Work out the finished part from the listing and answer in its coordinate system (mm). A direction names the side the tool comes from. Coordinates: 2 decimals unless noted, no trailing zeros. Loops run counter-clockwise (first coordinate to the right, second up) from the corner with the lowest first, then second, coordinate; pieces in that order, holes last. Notation, with made-up numbers: (-17, 37.5) -> (38, 37.5) arc R24 ccw to (38, 60.5) -> close; hole circle Ø11 at (23.25, -28.5). An arc over 180 degrees is marked (long way). Use a Markdown table: item, result.
Autodesk Inventor part; units mm, degrees
ref_plane "YZ Plane" through (0, 0, 0) normal (1, 0, 0) x (0, 1, 0)
ref_plane "XZ Plane" through (0, 0, 0) normal (0, 1, 0) x (-1, 0, 0)
ref_plane "XY Plane" through (0, 0, 0) normal (0, 0, 1) x (1, 0, 0)
sketch "Sketch1" plane through (0, 0, 0) normal (0, 0, 1) x (1, 0, 0)
  line L0 (0, 0) -> (15.75, 0)
  line L1 (15.75, 0) -> (15.75, -4)
  line L2 (0, -4) -> (0, 0)
  line L3 (17.65, -4) -> (17.65, -6)
  line L4 (-1.9, -6) -> (-1.9, -4)
  line L5 (-1.9, -4) -> (0, -4)
  line L6 (15.75, -4) -> (17.65, -4)
  line L7 (2, 0) -> (2, -6) construction
  line L8 (13.75, 0) -> (13.75, -6) construction
  arc A0 (13.75, -6) -> (2, -6) centre (7.875, -14.0922) ccw
  line L9 (17.65, -6) -> (13.75, -6)
  line L10 (2, -6) -> (-1.9, -6)
  dimension "d2" = 1.9
  dimension "d3" = 4
  dimension "d4" = 2
  dimension "d5" = 15.75
  dimension "d6" = 2
  dimension "d7" = 2
  dimension "d8" = 10
extrude "Extrusion1" add sketch "Sketch1" along normal blind 2.2
sketch "Sketch2" plane through (0, 0, 2.2) normal (0, 0, 1) x (1, 0, 0)
  line L0 (0, 0) -> (0.375, 0)
  line L1 (0.375, 0) -> (0.375, -4)
  line L2 (0.375, -4) -> (0, -4)
  line L3 (0, -4) -> (0, 0)
  line L4 (15.75, 0) -> (0, 0)
  line L5 (15.75, 0) -> (15.375, 0)
  line L6 (15.375, 0) -> (15.375, -4)
  line L7 (15.375, -4) -> (15.75, -4)
  line L8 (15.75, -4) -> (15.75, 0)
  dimension "d11" = 15
  dimension "d12" = 4
extrude "Extrusion2" cut sketch "Sketch2" against normal up to surface (2.2 mm away)
properties part number "Light Pipe modern"
Q1. Section B-B on y = -5 is taken. Determine the outline of the cut face in (x, z), and give its area (3 significant figures).
Solved:
| item | result |
|---|---|
| outline | (-1.9, 0) -> (3.71, 0) -> (3.71, 2.2) -> (-1.9, 2.2) -> close; (12.04, 0) -> (17.65, 0) -> (17.65, 2.2) -> (12.04, 2.2) -> close |
| area | 24.7 mm² |
Q2. Consider line 1 (X direction, y = -3.75, z = 1.4) (3 decimals); line 2 (Y direction, x = -0.5, z = 1); line 3 (X direction, y = -5.5, z = 0.25). Determine where each line is inside the solid, lowest interval first. Write a range as [from, to].
Solved:
| item | result |
|---|---|
| line 1 | [0.375, 15.375] |
| line 2 | [-6, -4] |
| line 3 | [-1.9, 2.76], [12.99, 17.65] |
Q3. Section D-D on x = 9.5 is taken. Determine the outline of the cut face in (y, z), and give its area (3 significant figures).
Solved:
| item | result |
|---|---|
| outline | (-4.23, 0) -> (0, 0) -> (0, 2.2) -> (-4.23, 2.2) -> close |
| area | 9.30 mm² |
Q4. For faces 1 (the flat face through (15.375, -2, 1)), 2 (the flat face through (-1, -4, 1)), 3 (the flat face through (17.65, -5, 1)), determine the directions among +Z, -Z, +X, -X, +Y, -Y from which every point of the face is accessible in a straight line to the end or side of a thin tool.
Solved:
| item | result |
|---|---|
| face 1 | +Z, -Z, +X, +Y |
| face 2 | +Z, -Z, -X, +Y |
| face 3 | +Z, -Z, +X, +Y, -Y |
Q5. Section A-A on z = 0.6 is taken. Determine the outline of the cut face in (x, y) (3 decimals), and give its area (3 significant figures).
Solved:
| item | result |
|---|---|
| outline | (-1.9, -6) -> (2, -6) arc R10 cw to (13.75, -6) -> (17.65, -6) -> (17.65, -4) -> (15.375, -4) -> (15.375, 0) -> (0.375, 0) -> (0.375, -4) -> (-1.9, -4) -> close |
| area | 83.8 mm² |
Q6. Given pin 1 Ø0.7 at (x, z) = (16.5, 0.5) entering from +Y; pin 2 Ø0.7 at (y, z) = (-2, 1) entering from +X (3 decimals), each flat-ended and moving along its own axis, determine where each tip first touches the part or whether it passes through.
Solved:
| item | result |
|---|---|
| pin 1 | y = -4 |
| pin 2 | x = 15.375 |
Q7. Section C-C on y = -1.5 is taken. Determine the outline of the cut face in (x, z) (3 decimals).
Solved:
| item | result |
|---|---|
| outline | (0.375, 0) -> (15.375, 0) -> (15.375, 2.2) -> (0.375, 2.2) -> close |
